Source: CAD feature listing. Evaluate the final solid. Frame: model axes, mm. A direction names the side the tool comes from. Round coordinates to 2 decimals unless told otherwise and drop trailing zeros. Order: outer loops, then holes, each group sorted by start corner. A loop starts at its lowest first (then second) coordinate and runs counter-clockwise, first axis right, second up. Notation, with made-up numbers: M -18,59 L 5,59 A24 cw 5,81 Z; hole C 9.5,32 d4. An arc over 180 degrees is marked long. Answer in a Markdown table with one row per item. Add a question column.
Autodesk Inventor part; units mm, degrees
ref_plane "YZ Plane" through (0, 0, 0) normal (1, 0, 0) x (0, 1, 0)
ref_plane "XZ Plane" through (0, 0, 0) normal (0, 1, 0) x (-1, 0, 0)
ref_plane "XY Plane" through (0, 0, 0) normal (0, 0, 1) x (1, 0, 0)
sketch "Sketch1" plane through (0, 0, 0) normal (0, 0, 1) x (1, 0, 0)
  circle A0 centre (0, 0) radius 2
  dimension "Diameter" = 4
extrude "Extrusion1" add sketch "Sketch1" along normal blind 12
sketch "Sketch2" plane through (0, 0, 12) normal (0, 0, 1) x (1, 0, 0)
  circle A0 centre (0, 0) radius 2
  circle A1 centre (0, 0) radius 3.5
  dimension "Head_Diameter" = 7
extrude "Extrusion2" add sketch "Sketch2" along normal blind 4 contours A0 | A1
sketch "Sketch3" plane through (0, 0, 16) normal (0, 0, 1) x (1, 0, 0)
  circle A0 centre (0, 0) radius 3.5
  circle A1 centre (0, 0) radius 1.7321 construction
  line L0 (0, 1.7321) -> (1.5, 0.866)
  line L1 (1.5, -0.866) -> (1.5, 0.866)
  line L2 (0, 1.7321) -> (-1.5, 0.866)
  line L3 (-1.5, -0.866) -> (-1.5, 0.866)
  line L4 (-1.5, -0.866) -> (0, -1.7321)
  line L5 (1.5, -0.866) -> (0, -1.7321)
  dimension "Hex_Width" = 3
extrude "Extrusion3" cut sketch "Sketch3" against normal blind 2 contours L0 L1 L5 L4 L3 L2
thread "Thread1"
chamfer "Chamfer1" distance 0.4 angle 45 2 edges at (-3.5, 0, 16) (-2, 0, 0)
equation "\"d9\" = ThreadLength"
equation "\"d12\" = Chamfer"
equation "\"ThreadLength\" = 20"
properties part number "SCREW, SOCKET HD, P, 12_9, M4X0_7X12" material "Steel, MS"
(1) Cut plane B-B (z = 13.75). Return loops of the section in (x, y), and give its area (3 significant figures).
(2) Cut plane C-C (z = 9.25). Return loops of the section in (x, y).
(3) Draft query along X for faces 1 (the face through (0, 0, 14)), 2 (the face through (0, 2, 6)), 3 (the face through (0, 0, 0)), 4 (the face through (0.74, 1.305, 15.014)). Return one class per face: +X half, -X half, draft (parallel to the pull), parting line (faces both ways), or undercut.
(4) Access query for faces 5 (the face through (2, -2, 12)), 6 (the face through (1.5, 0, 15)), 7 (the face through (3.233, 1.341, 13.775)). Directions: +Z, -Z, +X, -X, +Y, -Y. A direction counts if a zero-diameter tool reaches every point of the face in a straight line with its end or side. Return the directions, or none.
(5) Cut plane A-A (y = 0). Return loops of the section in (x, z).
(6) Line query: line 1 (X direction, y = -1, z = 5.25); line 2 (Y direction, x = -0.5, z = 14.75); line 3 (Z direction, x = 0, y = -3). Output: solid intervals per line, ascending. Write a range as from..to.
(7) Pin query (flat end, axial travel): pin 1 (0.9 mm diameter, centred on x = 0, y = 0.5, fed in from +Z); pin 2 (1 mm diameter, centred on x = 2, z = 14.5, fed in from +Y). Return the tip coordinate at first contact, or that it passes through.
Answer list:
| question | item | result |
|---|---|---|
| 1 | outline | C 0,0 d7 |
| 1 | area | 38.5 mm² |
| 2 | outline | C 0,0 d4 |
| 3 | face 1 | undercut |
| 3 | face 2 | parting line |
| 3 | face 3 | draft |
| 3 | face 4 | undercut |
| 4 | face 5 | -Z |
| 4 | face 6 | +Z |
| 4 | face 7 | +Z, -Z |
| 5 | outline | M -3.5,12 L -2,12 L -2,0.4 L -1.6,0 L 1.6,0 L 2,0.4 L 2,12 L 3.5,12 L 3.5,15.6 L 3.1,16 L 1.5,16 L 1.5,14 L -1.5,14 L -1.5,16 L -3.1,16 L -3.5,15.6 Z |
| 6 | line 1 | -1.73..1.73 |
| 6 | line 2 | -3.46..-1.44, 1.44..3.46 |
| 6 | line 3 | 12..16 |
| 7 | pin 1 | z = 14 |
| 7 | pin 2 | y = 3.16 |
